Design review of the part built by this model. Coordinates are the model's own, in mm. Face numbers are marked on the shaded views. A direction names the side the tool comes from. Coordinates: 2 decimals unless noted, no trailing zeros. Loops run counter-clockwise (first coordinate to the right, second up) from the corner with the lowest first, then second, coordinate; pieces in that order, holes last. Notation, with made-up numbers: (-8.5, -35) - (20.5, -35) arc R16 cw to (20.5, -4) - close; hole circle Ø1 at (69, 23.25). An arc over 180 degrees is marked (long way). Return JSON: item names as keys, results as strings. Group by question number.
from build123d import *

# Parameters (mm, degrees)
ESQUISSE1_W             = 113
ESQUISSE1_H             = 13
ESQUISSE1_R             = 1.6
BOSS_EXTRU_1_DEPTH      = 1
ESQUISSE2_W             = 113
ESQUISSE2_H             = 1
BOSS_EXTRU_2_DEPTH      = 9
ENL_V_MAT_EXTRU_1_REACH = 116.184
ESQUISSE3_R             = 1.6


with BuildPart() as part:
    # Esquisse1 → Boss.-Extru.1 (new body)
    with BuildSketch(Plane(origin=(0, 0, 0), x_dir=(1, 0, 0), z_dir=(0, 1, 0))):
        with Locations((56.5, 6.5)):
            Rectangle(ESQUISSE1_W, ESQUISSE1_H)
        with Locations(Location((79, 6.5, 0), (0, 0, 270))):
            Circle(ESQUISSE1_R, mode=Mode.SUBTRACT)
        with Locations(Location((29.5, 6.5, 0), (0, 0, 270))):
            Circle(ESQUISSE1_R, mode=Mode.SUBTRACT)
    extrude(amount=BOSS_EXTRU_1_DEPTH)

    # Esquisse2 → Boss.-Extru.2 (add)
    with BuildSketch(Plane(origin=(0, 1, 0), x_dir=(1, 0, 0), z_dir=(0, 1, 0))):
        with Locations((56.5, 12.5)):
            Rectangle(ESQUISSE2_W, ESQUISSE2_H)
        with Locations((56.5, 0.5)):
            Rectangle(ESQUISSE2_W, ESQUISSE2_H)
    extrude(amount=BOSS_EXTRU_2_DEPTH)

    # Esquisse3 → Enlèv. mat.-Extru.1 (cut, up to next)
    with BuildSketch(Plane.XY, mode=Mode.PRIVATE) as enl_v_mat_extru_1_sk1:
        with Locations((99.4, 5)):
            Circle(ESQUISSE3_R)
    enl_v_mat_extru_1_tool1 = extrude(enl_v_mat_extru_1_sk1.sketch, amount=-ENL_V_MAT_EXTRU_1_REACH, mode=Mode.PRIVATE) & part.part
    # Esquisse3 → Enlèv. mat.-Extru.1 (cut, up to next)
    with BuildSketch(Plane.XY, mode=Mode.PRIVATE) as enl_v_mat_extru_1_sk2:
        with Locations((61.8, 5)):
            Circle(ESQUISSE3_R)
    enl_v_mat_extru_1_tool2 = extrude(enl_v_mat_extru_1_sk2.sketch, amount=-ENL_V_MAT_EXTRU_1_REACH, mode=Mode.PRIVATE) & part.part
    # Esquisse3 → Enlèv. mat.-Extru.1 (cut, up to next)
    with BuildSketch(Plane.XY, mode=Mode.PRIVATE) as enl_v_mat_extru_1_sk3:
        with Locations((24.2, 5)):
            Circle(ESQUISSE3_R)
    enl_v_mat_extru_1_tool3 = extrude(enl_v_mat_extru_1_sk3.sketch, amount=-ENL_V_MAT_EXTRU_1_REACH, mode=Mode.PRIVATE) & part.part
    add(enl_v_mat_extru_1_tool1.solids().sort_by_distance((99.4, 5, 0))[0], mode=Mode.SUBTRACT)
    add(enl_v_mat_extru_1_tool2.solids().sort_by_distance((61.8, 5, 0))[0], mode=Mode.SUBTRACT)
    add(enl_v_mat_extru_1_tool3.solids().sort_by_distance((24.2, 5, 0))[0], mode=Mode.SUBTRACT)


solid = part.part
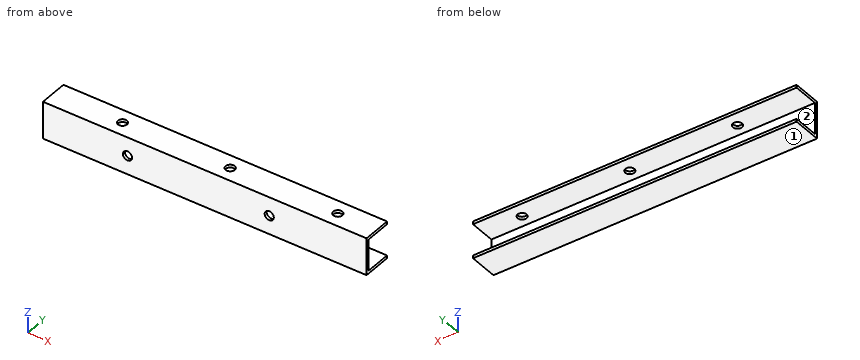
Item 1: Add section D-D (x = 67.5). State the section outline as (y, z) points.
Item 2: For the marked faces 1 and 2, list the 3-axis set-ups (+Z, -Z, +X, -X, +Y, -Y) from which the entire face can be reached by the end or side of a thin tool; tool diameter is ignored.
Item 3: Add section A-A (z = -6.5). State the section outline as (x, y) points.
Item 4: For P1, Ø2.5, axis at x = 61.8, y = 5, coming from the +Z side; P2, Ø5, axis at y = 6, z = -9, coming from the +X side, all flat-tipped, find the tip position at first contact; note any pin that passes through.
Item 5: Add section C-C (x = 24.2). State the section outline as (y, z) points.
Item 6: Add section B-B (y = 5). State the section outline as (x, z) points.
Item 7: To check wall thickness, follow line 1 (Z direction, x = 50, y = 7); line 2 (X direction, y = 0.3, z = -6.5); line 3 (Y direction, x = 61.8, z = -0.75). State the ranges of each line that lie inside material, in increasing order. Write a range as from..to.
Answers below:
{
 "1": {"outline": "(0, -13) - (10, -13) - (10, -12) - (1, -12) - (1, -1) - (10, -1) - (10, 0) - (0, 0) - close"},
 "2": {"face 1": "-Z, +X, -X, +Y, -Y", "face 2": "+X, -X, +Y"},
 "3": {"outline": "(0, 0) - (27.9, 0) - (27.9, 1) - (0, 1) - close; (31.1, 0) - (77.4, 0) - (77.4, 1) - (31.1, 1) - close; (80.6, 0) - (113, 0) - (113, 1) - (80.6, 1) - close"},
 "4": {"P1": "stops at z = -12", "P2": "passes through"},
 "5": {"outline": "(0, -13) - (10, -13) - (10, -12) - (1, -12) - (1, -1) - (3.4, -1) - (3.4, 0) - (0, 0) - close; (6.6, -1) - (10, -1) - (10, 0) - (6.6, 0) - close"},
 "6": {"outline": "(0, -13) - (113, -13) - (113, -12) - (0, -12) - close; (0, -1) - (22.6, -1) - (22.6, 0) - (0, 0) - close; (25.8, -1) - (60.2, -1) - (60.2, 0) - (25.8, 0) - close; (63.4, -1) - (97.8, -1) - (97.8, 0) - (63.4, 0) - close; (101, -1) - (113, -1) - (113, 0) - (101, 0) - close"},
 "7": {"line 1": "z = -13..-12, -1..0", "line 2": "x = 0..27.9, 31.1..77.4, 80.6..113", "line 3": "y = 0..3.4, 6.6..10"}
}
